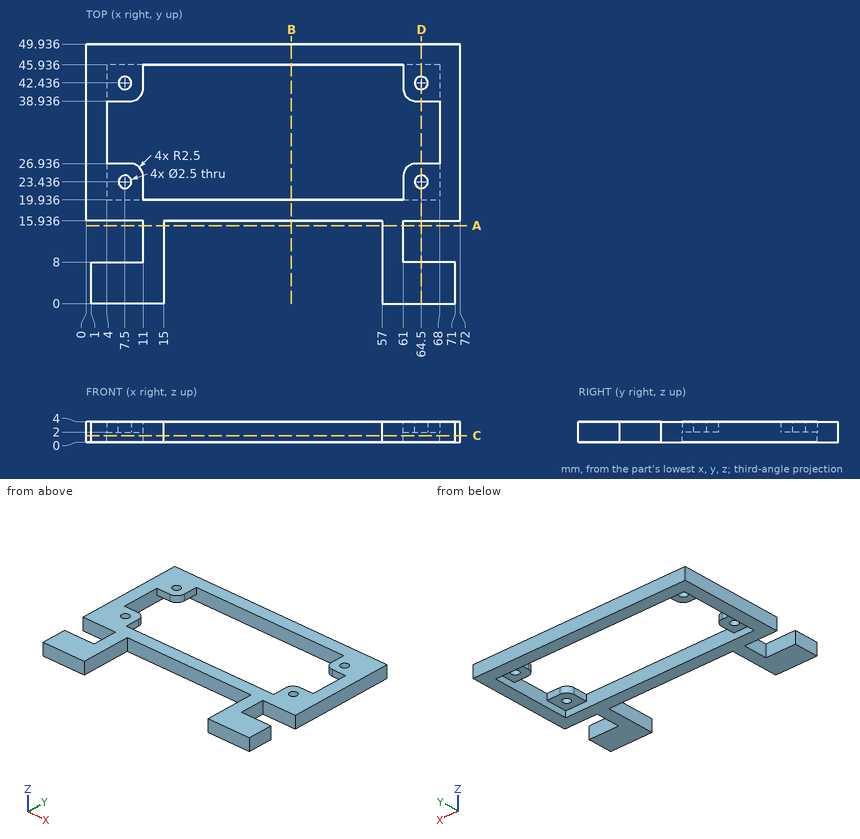
Geometry check sheet. Reference: drawing and pictorial views, mm from the part's lowest x, y, z. Round coordinates to 2 decimals unless told otherwise and drop trailing zeros. Write each loop counter-clockwise with the first axis right and the second up, starting at its lowest first coordinate (ties: lowest second). Pieces come first, ordered by that corner, then holes.
Item 1: Section check B-B (x = 39.5). Record the boundary of the cut face in (y, z).
Determined:
outline: (15.94, 0) - (19.94, 0) - (19.94, 4) - (15.94, 4) - close; (45.94, 0) - (49.94, 0) - (49.94, 4) - (45.94, 4) - close
Item 2: Section check A-A (y = 15). Record the boundary of the cut face in (x, z), plus the area to 3 significant figures.
Determined:
outline: (11, 0) - (15, 0) - (15, 4) - (11, 4) - close; (57, 0) - (61, 0) - (61, 4) - (57, 4) - close
area: 32.0 mm2
Item 3: Section check C-C (z = 1.3). Record the boundary of the cut face in (x, y).
Determined:
outline: (0, 15.94) - (11, 15.94) - (11, 8) - (1, 8) - (1, 0) - (15, 0) - (15, 15.94) - (57, 15.94) - (57, 0) - (71, 0) - (71, 8) - (61, 8) - (61, 15.94) - (72, 15.94) - (72, 49.94) - (0, 49.94) - close; hole (4, 19.94) - (68, 19.94) - (68, 45.94) - (4, 45.94) - close
Item 4: Material ranges on line 1 along Y through (x, z) = (65.5, 0.6); line 2 along X through (y, z) = (32, 1.05); line 3 along X through (y, z) = (7.5, 2), recorded low to high.
Determined:
line 1: y = 0 to 8, 15.94 to 19.94, 45.94 to 49.94
line 2: x = 0 to 4, 68 to 72
line 3: x = 1 to 15, 57 to 71
Item 5: Section check D-D (x = 64.5). Record the boundary of the cut face in (y, z).
Determined:
outline: (0, 0) - (8, 0) - (8, 4) - (0, 4) - close; (15.94, 0) - (19.94, 0) - (19.94, 2) - (22.19, 2) - (22.19, 4) - (15.94, 4) - close; (24.69, 2) - (26.94, 2) - (26.94, 4) - (24.69, 4) - close; (38.94, 2) - (41.19, 2) - (41.19, 4) - (38.94, 4) - close; (43.69, 2) - (45.94, 2) - (45.94, 0) - (49.94, 0) - (49.94, 4) - (43.69, 4) - close
Item 6: Go/stop test with flat-tipped pins: pin 1 Ø2 at (x, y) = (6, 24.5) entering from -Z; pin 2 Ø1.2 at (x, z) = (31.5, 2.5) entering from -Y; pin 3 Ø2 at (x, y) = (44.5, 21) entering from -Z; pin 4 Ø1.2 at (y, z) = (5.5, 2.5) entering from +X. Record where each tip stops, or that it passes through.
Determined:
pin 1: stops at z = 2
pin 2: stops at y = 15.94
pin 3: passes through
pin 4: stops at x = 71
